Input: part model. Units: mm. Frame: model coordinates. A direction names the side the tool comes from. Coordinates: 2 decimals unless noted, no trailing zeros. Order: outer loops, then holes, each group sorted by start corner. A loop starts at its lowest first (then second) coordinate and runs counter-clockwise, first axis right, second up. Notation, with made-up numbers: (-27, -22) - (-20, -22) arc R21 cw to (-20, 16) - close; hole circle Ø8 at (47, -30.75). An arc over 180 degrees is marked (long way). Use a Markdown table: item, result. Add a question column.
from build123d import *

# Parameters (mm, degrees)
SKETCH1_W           = 42
SKETCH1_H           = 42
BOSS_EXTRUDE1_DEPTH = 32
SKETCH2_R           = 11
BOSS_EXTRUDE2_DEPTH = 2
SKETCH3_R           = 2.5
BOSS_EXTRUDE3_DEPTH = 22
SKETCH4_R           = 1.5
CUT_EXTRUDE1_DEPTH  = 5
CHAMFER1_SIZE       = 5


with BuildPart() as part:
    # Sketch1 → Boss-Extrude1 (new body)
    with BuildSketch(Plane(origin=(0, 0, 0), x_dir=(1, 0, 0), z_dir=(0, 1, 0))):
        Rectangle(SKETCH1_W, SKETCH1_H)
    extrude(amount=BOSS_EXTRUDE1_DEPTH)

    # Sketch2 → Boss-Extrude2 (add)
    with BuildSketch(Plane(origin=(0, 32, 0), x_dir=(1, 0, 0), z_dir=(0, 1, 0))):
        with Locations(Location((0, 0, 0), (0, 0, 270))):
            Circle(SKETCH2_R)
    extrude(amount=BOSS_EXTRUDE2_DEPTH)

    # Sketch3 → Boss-Extrude3 (add)
    with BuildSketch(Plane(origin=(0, 34, 0), x_dir=(1, 0, 0), z_dir=(0, 1, 0))):
        with Locations(Location((0, 0, 0), (0, 0, 270))):
            Circle(SKETCH3_R)
    extrude(amount=BOSS_EXTRUDE3_DEPTH)

    # Sketch4 → Cut-Extrude1 (cut)
    with BuildSketch(Plane(origin=(0, 32, 0), x_dir=(1, 0, 0), z_dir=(0, 1, 0))):
        with Locations(Location((15.5, 15.5, 0), (0, 0, 270))):
            Circle(SKETCH4_R)
        with Locations(Location((15.5, -15.5, 0), (0, 0, 270))):
            Circle(SKETCH4_R)
        with Locations(Location((-15.5, -15.5, 0), (0, 0, 270))):
            Circle(SKETCH4_R)
        with Locations(Location((-15.5, 15.5, 0), (0, 0, 270))):
            Circle(SKETCH4_R)
    extrude(amount=-CUT_EXTRUDE1_DEPTH, mode=Mode.SUBTRACT)

    # Chamfer1
    chamfer1_edges = [part.edges().sort_by_distance(p)[0] for p in [
        (21, 16, 21),
        (-21, 16, 21),
        (-21, 16, -21),
        (21, 16, -21),
    ]]
    chamfer(chamfer1_edges, length=CHAMFER1_SIZE)


solid = part.part
1) Reachability of faces 1 (the flat face through (19, 16, 18)), 2 (the flat face through (-15, 27, -16)) from +Z, -Z, +X, -X, +Y, -Y: full face, straight path, thin tool, end or side. Return the list, or none.
2) Cut plane B-B (y = 11.5). Return the cut outline in (x, z).
3) Material intervals for L1, parallel to X at y = 30, z = 15.5; L2, parallel to Y at x = -1, z = -7; L3, parallel to Y at x = 13, z = 6, sorted ascending.
4) Cut plane D-D (y = 50). Return the cut outline in (x, z), and give its area (3 significant figures).
5) Cut plane A-A (x = 0). Return the cut outline in (y, z).
6) Pull-direction query (X, two-part tool) for faces 3 (the flat face through (0, 16, -21)), 4 (the flat face through (-18, 16, -19)), 5 (the flat face through (16, 27, 15)), 6 (the flat face through (19, 16, -18)); classes: pulls with the +X half, pulls with the -X half, needs draft (parallel to the pull), parting line crosses it, or undercut.
7) Cut plane C-C (z = -9). Return the cut outline in (x, y).
8) Contact query for flat-ended pins moving along their axis: P1, Ø5, axis at x = 15.5, z = 15.5, coming from the +Y side; P2, Ø12, axis at x = -1, z = 16.5, coming from the +Y side; P3, Ø0.9, axis at x = 16, z = -15.5, coming from the +Y side. Output: stop coordinate, or through.
Computed:
| question | item | result |
|---|---|---|
| 1 | face 1 | +Z, +X, +Y, -Y |
| 1 | face 2 | +Y |
| 2 | outline | (-21, -16) - (-16, -21) - (16, -21) - (21, -16) - (21, 16) - (16, 21) - (-16, 21) - (-21, 16) - close |
| 3 | L1 | x = -21 to -17, -14 to 14, 17 to 21 |
| 3 | L2 | y = 0 to 34 |
| 3 | L3 | y = 0 to 32 |
| 4 | outline | circle Ø5 at (0, 0) |
| 4 | area | 19.6 mm2 |
| 5 | outline | (0, -21) - (32, -21) - (32, -11) - (34, -11) - (34, -2.5) - (56, -2.5) - (56, 2.5) - (34, 2.5) - (34, 11) - (32, 11) - (32, 21) - (0, 21) - close |
| 6 | face 3 | needs draft |
| 6 | face 4 | pulls with the -X half |
| 6 | face 5 | undercut |
| 6 | face 6 | pulls with the +X half |
| 7 | outline | (-21, 0) - (21, 0) - (21, 32) - (6.32, 32) - (6.32, 34) - (-6.32, 34) - (-6.32, 32) - (-21, 32) - close |
| 8 | P1 | stops at y = 32 |
| 8 | P2 | stops at y = 34 |
| 8 | P3 | stops at y = 27 |
